Can you work these out from the model? Positions are in its coordinate system, mm. A direction names the side the tool comes from. Round coordinates to 2 decimals unless told otherwise and drop trailing zeros. Order: outer loops, then holes, each group sorted by start corner. A loop starts at its lowest first (then second) coordinate and runs counter-clockwise, first axis right, second up. Notation, with made-up numbers: (57.25, 64.25) -> (109.25, 64.25) arc R27 cw to (109.25, 89.25) -> close; hole circle Ø11 at (21, -15). An arc over 180 degrees is marked (long way). Use a Markdown table: item, result. Add a question column.
Q1. I need wall thicknesses on line 1 along X through (y, z) = (-31, 0.5); line 2 along X through (y, z) = (-40, 1.3); line 3 along Y through (x, z) = (12, 4.1). Which ranges of each line are inside material? Lowest first, please. Write a range as [from, to].
Q2. If we section it at C-C on z = 4.1: Give the number of separate pieces and of enclosed holes in the cut face, plus the area to 3 significant figures.
Q3. I'm going to push flat-ended pins straight in: pin 1 Ø2 at (x, y) = (13, -31.5) entering from -Z; pin 2 Ø1 at (x, y) = (45.5, -13.5) entering from +Z; pin 3 Ø5.5 at (x, y) = (-23, 43) entering from -Z. Where does each tip first touch, or does it pass through?
Q4. We'd pull the mould along Y, two halves only. Please class faces 5 (the face through (-22, 41, 2)), 6 (the face through (-39, -2, 5)), 7 (the face through (13, -4, 3)), 8 (the face through (80.2, 20.06, 2.46)): +Y half, -Y half, draft (parallel to the pull), parting line (faces both ways), or undercut.
Q5. If we section it at D-D on y = -50: List the corners of the cut face in (x, z) for me, plus the area to 3 significant figures.
Q6. If we section it at A-A on y = -26: List the corners of the cut face in (x, z) for me.
Q7. If we section it at B-B on x = 5.5: List the corners of the cut face in (y, z) for me.
Q8. For faces 1 (the face through (24.22, -78.78, 2.46)), 2 (the face through (-68, 18, 3)), 3 (the face through (-34, 71, 3)), 4 (the face through (0, -58, 1.5)), which set-ups out of +Z, -Z, +X, -X, +Y, -Y let a thin tool reach every point of the face, with its end or its side?
```python
from build123d import *

# Parameters (mm, degrees)
EXTRUDE_2156_DEPTH      = 5
FILLET_3_R              = 1.5
FILLET_4_R              = 1.5
FILLET_5_R              = 1.5
FILLET_6_R              = 1.5
FILLET_8_R              = 1.5
FILLET_9_R              = 1.5
FILLET_10_R             = 1
SKETCH_5_R              = 1.5
CUT_EXTRUDE_4477_DEPTH  = 2
SKETCH_12_R             = 3.5
CUT_EXTRUDE_5428_DEPTH  = 3
CUT_EXTRUDE_START       = -3.5
CUT_EXTRUDE_6211_DEPTH  = 3.5
SKETCH_8_W              = 26
SKETCH_8_H              = 49
CUT_EXTRUDE_6713_DEPTH  = 5
SKETCH_9_R              = 1.5
CUT_EXTRUDE_7322_DEPTH  = 2
SKETCH_10_R             = 3.5
CUT_EXTRUDE_8110_DEPTH  = 3
SKETCH_11_R             = 1.5
CUT_EXTRUDE_8691_DEPTH  = 5
SKETCH_14_W             = 68
SKETCH_14_H             = 4
CUT_EXTRUDE_8943_DEPTH  = 10
SKETCH_15_R             = 1
CUT_EXTRUDE_9740_DEPTH  = 4
SKETCH_16_R             = 1
CUT_EXTRUDE_10725_DEPTH = 4
SKETCH_17_R             = 1
CUT_EXTRUDE_11590_DEPTH = 4
SKETCH_18_R             = 3.5
CUT_EXTRUDE_12205_DEPTH = 2
SKETCH_19_W             = 68
SKETCH_19_H             = 11
CUT_EXTRUDE_3_DEPTH     = 5


with BuildPart() as part:
    # 草图1 → Extrude 2156 (new body)
    with BuildSketch(Plane.XY):
        with BuildLine():
            Line((40.572949017, 63.247239682), (56.631189606, 41.14496766))
            Line((56.631189606, 41.14496766), (72.029031786, 19.951656069))
            ThreePointArc((72.029031786, 19.951656069), (73.431066875, 18.895554003), (75.184005217, 18.804663237))
            Line((75.184005217, 18.804663237), (86.825399574, 21.716353029))
            ThreePointArc((86.825399574, 21.716353029), (88.776371499, -11.358074817), (78.561436026, -42.875992928))
            Line((78.561436026, -42.875992928), (68.669508852, -37.477336526))
            ThreePointArc((68.669508852, -37.477336526), (66.987138464, -37.120716922), (65.385340306, -37.74664849))
            Line((65.385340306, -37.74664849), (43.096303273, -55.160752752))
            Line((43.096303273, -55.160752752), (23.649832714, -70.354000687))
            ThreePointArc((23.649832714, -70.354000687), (22.63495231, -71.818183128), (22.6292966, -73.599693854))
            Line((22.6292966, -73.599693854), (26.30288371, -85.547696103))
            ThreePointArc((26.30288371, -85.547696103), (0, -89.5), (-26.30288371, -85.547696103))
            Line((-26.30288371, -85.547696103), (-22.6292966, -73.599693854))
            ThreePointArc((-22.6292966, -73.599693854), (-22.63495231, -71.818183128), (-23.649832714, -70.354000687))
            Line((-23.649832714, -70.354000687), (-43.096303273, -55.160752752))
            Line((-43.096303273, -55.160752752), (-65.385340306, -37.74664849))
            ThreePointArc((-65.385340306, -37.74664849), (-66.987138464, -37.120716922), (-68.669508852, -37.477336526))
            Line((-68.669508852, -37.477336526), (-78.561436026, -42.875992928))
            ThreePointArc((-78.561436026, -42.875992928), (-88.776371499, -11.358074817), (-86.825399574, 21.716353029))
            Line((-86.825399574, 21.716353029), (-75.184005217, 18.804663237))
            ThreePointArc((-75.184005217, 18.804663237), (-73.431066875, 18.895554003), (-72.029031786, 19.951656069))
            Line((-72.029031786, 19.951656069), (-56.631189606, 41.14496766))
            Line((-56.631189606, 41.14496766), (-40.572949017, 63.247239682))
            ThreePointArc((-40.572949017, 63.247239682), (-40.146830451, 64.083544456), (-40, 65.010595439))
            Line((-40, 65.010595439), (-40, 74))
            Line((-40, 74), (-40, 80.06403687))
            Line((-40, 80.06403687), (-34, 82.790397994))
            Line((-34, 82.790397994), (-34, 77))
            Line((-34, 77), (34, 77))
            Line((34, 77), (34, 82.790397994))
            Line((34, 82.790397994), (40, 80.06403687))
            Line((40, 80.06403687), (40, 74))
            Line((40, 74), (40, 65.010595439))
            ThreePointArc((40, 65.010595439), (40.146830451, 64.083544456), (40.572949017, 63.247239682))
        make_face()
    extrude(amount=EXTRUDE_2156_DEPTH)

    # 圆角3
    fillet_3_edges = [part.edges().sort_by_distance(p)[0] for p in [
        (78.561436026, -42.875992928, 2.5),
    ]]
    fillet(fillet_3_edges, radius=FILLET_3_R)

    # 圆角4
    fillet_4_edges = [part.edges().sort_by_distance(p)[0] for p in [
        (26.30288371, -85.547696103, 2.5),
    ]]
    fillet(fillet_4_edges, radius=FILLET_4_R)

    # 圆角5
    fillet_5_edges = [part.edges().sort_by_distance(p)[0] for p in [
        (-26.30288371, -85.547696103, 2.5),
    ]]
    fillet(fillet_5_edges, radius=FILLET_5_R)

    # 圆角6
    fillet_6_edges = [part.edges().sort_by_distance(p)[0] for p in [
        (-78.561436026, -42.875992928, 2.5),
    ]]
    fillet(fillet_6_edges, radius=FILLET_6_R)

    # 圆角8
    fillet_8_edges = [part.edges().sort_by_distance(p)[0] for p in [
        (86.825399574, 21.716353029, 2.5),
    ]]
    fillet(fillet_8_edges, radius=FILLET_8_R)

    # 圆角9
    fillet_9_edges = [part.edges().sort_by_distance(p)[0] for p in [
        (-86.825399574, 21.716353029, 2.5),
    ]]
    fillet(fillet_9_edges, radius=FILLET_9_R)

    # 圆角10
    fillet_10_edges = [part.edges().sort_by_distance(p)[0] for p in [
        (-40, 80.06403687, 2.5),
        (-34, 82.790397994, 2.5),
        (34, 82.790397994, 2.5),
        (40, 80.06403687, 2.5),
    ]]
    fillet(fillet_10_edges, radius=FILLET_10_R)

    # 草图5 → Cut-Extrude 4477 (cut)
    with BuildSketch(Plane.XY.offset(5)):
        with Locations((47.738500848, 48.280798842)):
            Circle(SKETCH_5_R)
        with Locations((68.310984678, 19.965204039)):
            Circle(SKETCH_5_R)
        with Locations(Location((-68.310984678, 19.965204039, 0), (0, 0, 180))):
            Circle(SKETCH_5_R)
        with Locations(Location((-47.738500848, 48.280798842, 0), (0, 0, 180))):
            Circle(SKETCH_5_R)
        with Locations((60.161576933, -38.020845084)):
            Circle(SKETCH_5_R)
        with Locations((32.581200557, -59.56899672)):
            Circle(SKETCH_5_R)
        with Locations(Location((-60.161576933, -38.020845084, 0), (0, 0, 180))):
            Circle(SKETCH_5_R)
        with Locations(Location((-32.581200557, -59.56899672, 0), (0, 0, 180))):
            Circle(SKETCH_5_R)
    extrude(amount=-CUT_EXTRUDE_4477_DEPTH, mode=Mode.SUBTRACT)

    # 草图12 → Cut-Extrude 5428 (cut)
    with BuildSketch(Plane(origin=(0, 0, 0), x_dir=(-1, 0, 0), z_dir=(0, 0, -1))):
        with Locations((47.738500848, 48.280798842)):
            Circle(SKETCH_12_R)
        with Locations((68.310984678, 19.965204039)):
            Circle(SKETCH_12_R)
        with Locations((-68.310984678, 19.965204039)):
            Circle(SKETCH_12_R)
        with Locations((-47.738500848, 48.280798842)):
            Circle(SKETCH_12_R)
        with Locations((32.581200557, -59.56899672)):
            Circle(SKETCH_12_R)
        with Locations((60.161576933, -38.020845084)):
            Circle(SKETCH_12_R)
        with Locations((13.527038551, -115.928745256)):
            Circle(SKETCH_12_R)
        with Locations((-60.161576933, -38.020845084)):
            Circle(SKETCH_12_R)
        with Locations((-32.581200557, -59.56899672)):
            Circle(SKETCH_12_R)
    extrude(amount=-CUT_EXTRUDE_5428_DEPTH, mode=Mode.SUBTRACT)

    # 草图7 → Cut-Extrude 6211 (cut)
    with BuildSketch(Plane.XY.offset(5).offset(CUT_EXTRUDE_START)):
        with BuildLine():
            Line((-8, 77), (-8, -89.141741064))
            ThreePointArc((-8, -89.141741064), (0, -89.5), (8, -89.141741064))
            Line((8, -89.141741064), (8, 77))
            Line((8, 77), (-8, 77))
        make_face()
    extrude(amount=CUT_EXTRUDE_6211_DEPTH, mode=Mode.SUBTRACT)

    # 草图8 → Cut-Extrude 6713 (cut)
    with BuildSketch(Plane.XY.offset(5)):
        with Locations((0, -3.5)):
            Rectangle(SKETCH_8_W, SKETCH_8_H)
    extrude(amount=-CUT_EXTRUDE_6713_DEPTH, mode=Mode.SUBTRACT)

    # 草图9 → Cut-Extrude 7322 (cut)
    with BuildSketch(Plane.XY.offset(5)):
        with Locations((12, 25)):
            Circle(SKETCH_9_R)
        with Locations(Location((-12, 25, 0), (0, 0, 180))):
            Circle(SKETCH_9_R)
        with Locations((-12, -32)):
            Circle(SKETCH_9_R)
        with Locations(Location((12, -32, 0), (0, 0, 180))):
            Circle(SKETCH_9_R)
    extrude(amount=-CUT_EXTRUDE_7322_DEPTH, mode=Mode.SUBTRACT)

    # 草图10 → Cut-Extrude 8110 (cut)
    with BuildSketch(Plane(origin=(0, 0, 0), x_dir=(-1, 0, 0), z_dir=(0, 0, -1))):
        with Locations((12, 25)):
            Circle(SKETCH_10_R)
        with Locations(Location((-12, 25, 0), (0, 0, 180))):
            Circle(SKETCH_10_R)
        with Locations(Location((12, -32, 0), (0, 0, 180))):
            Circle(SKETCH_10_R)
        with Locations((-12, -32)):
            Circle(SKETCH_10_R)
    extrude(amount=-CUT_EXTRUDE_8110_DEPTH, mode=Mode.SUBTRACT)

    # 草图11 → Cut-Extrude 8691 (cut)
    with BuildSketch(Plane.XY.offset(5)):
        with Locations((22.5, 57.8)):
            Circle(SKETCH_11_R)
        with Locations((22.5, 42.8)):
            Circle(SKETCH_11_R)
        with Locations(Location((-22.5, 42.8, 0), (0, 0, 180))):
            Circle(SKETCH_11_R)
        with Locations(Location((-22.5, 57.8, 0), (0, 0, 180))):
            Circle(SKETCH_11_R)
    extrude(amount=-CUT_EXTRUDE_8691_DEPTH, mode=Mode.SUBTRACT)

    # 草图14 → Cut-Extrude 8943 (cut)
    with BuildSketch(Plane(origin=(0, 0, 0), x_dir=(-1, 0, 0), z_dir=(0, 0, -1))):
        with Locations((0, 75)):
            Rectangle(SKETCH_14_W, SKETCH_14_H)
    extrude(amount=-CUT_EXTRUDE_8943_DEPTH, mode=Mode.SUBTRACT)

    # 草图15 → Cut-Extrude 9740 (cut)
    with BuildSketch(Plane.XY.offset(5)):
        with Locations(Location((-45.5, -13.5, 0), (0, 0, 180))):
            Circle(SKETCH_15_R)
        with Locations(Location((-34, 43, 0), (0, 0, 180))):
            Circle(SKETCH_15_R)
        with Locations((34, 43)):
            Circle(SKETCH_15_R)
        with Locations((45.5, -13.5)):
            Circle(SKETCH_15_R)
    extrude(amount=-CUT_EXTRUDE_9740_DEPTH, mode=Mode.SUBTRACT)

    # 草图16 → Cut-Extrude 10725 (cut)
    with BuildSketch(Plane.XY.offset(5)):
        with Locations((-70.6, -32.7)):
            Circle(SKETCH_16_R)
        with Locations((-70.6, 9.5)):
            Circle(SKETCH_16_R)
        with Locations((70.6, 9.5)):
            Circle(SKETCH_16_R)
        with Locations((70.6, -32.7)):
            Circle(SKETCH_16_R)
    extrude(amount=-CUT_EXTRUDE_10725_DEPTH, mode=Mode.SUBTRACT)

    # 草图17 → Cut-Extrude 11590 (cut)
    with BuildSketch(Plane.XY.offset(5)):
        with Locations((85.690046638, -3.237648509)):
            Circle(SKETCH_17_R)
        with Locations((85.690046638, -13.762351491)):
            Circle(SKETCH_17_R)
        with Locations((52.309953362, -13.762351491)):
            Circle(SKETCH_17_R)
        with Locations((52.309953362, -3.237648509)):
            Circle(SKETCH_17_R)
        with Locations(Location((-52.309953362, -13.762351491, 0), (0, 0, 180))):
            Circle(SKETCH_17_R)
        with Locations(Location((-85.690046638, -3.237648509, 0), (0, 0, 180))):
            Circle(SKETCH_17_R)
        with Locations(Location((-52.309953362, -3.237648509, 0), (0, 0, 180))):
            Circle(SKETCH_17_R)
        with Locations(Location((-85.690046638, -13.762351491, 0), (0, 0, 180))):
            Circle(SKETCH_17_R)
    extrude(amount=-CUT_EXTRUDE_11590_DEPTH, mode=Mode.SUBTRACT)

    # 草图18 → Cut-Extrude 12205 (cut)
    with BuildSketch(Plane(origin=(0, 0, 0), x_dir=(-1, 0, 0), z_dir=(0, 0, -1))):
        with Locations((-22.5, 57.8)):
            Circle(SKETCH_18_R)
        with Locations((-22.5, 42.8)):
            Circle(SKETCH_18_R)
        with Locations((22.5, 42.8)):
            Circle(SKETCH_18_R)
        with Locations((22.5, 57.8)):
            Circle(SKETCH_18_R)
    extrude(amount=-CUT_EXTRUDE_12205_DEPTH, mode=Mode.SUBTRACT)

    # 草图19 → 切除-拉伸3 (cut, symmetric)
    with BuildSketch(Plane.XY.offset(5)):
        with Locations((0, 67.5)):
            Rectangle(SKETCH_19_W, SKETCH_19_H)
    extrude(amount=CUT_EXTRUDE_3_DEPTH, both=True, mode=Mode.SUBTRACT)


solid = part.part
```
Answer below:
| question | item | result |
|---|---|---|
| 1 | line 1 | [-83.96, -15.35], [-8.65, 8.65], [15.35, 83.96] |
| 1 | line 2 | [-80.06, -73.29], [-57.27, 57.27], [73.29, 80.06] |
| 1 | line 3 | [-88.69, -33.5], [-30.5, -28], [21, 23.5], [26.5, 62] |
| 2 | separate pieces | 2 |
| 2 | enclosed holes | 32 |
| 2 | area | 15,900 mm² |
| 3 | pin 1 | z = 3 |
| 3 | pin 2 | z = 1 |
| 3 | pin 3 | z = 2 |
| 4 | face 5 | undercut |
| 4 | face 6 | draft |
| 4 | face 7 | undercut |
| 4 | face 8 | +Y half |
| 5 | outline | (-49.7, 0) -> (49.7, 0) -> (49.7, 5) -> (8, 5) -> (8, 1.5) -> (-8, 1.5) -> (-8, 5) -> (-49.7, 5) -> close |
| 5 | area | 441 mm² |
| 6 | outline | (-85.64, 0) -> (-13, 0) -> (-13, 5) -> (-85.64, 5) -> close; (13, 0) -> (85.64, 0) -> (85.64, 5) -> (13, 5) -> close |
| 7 | outline | (-89.33, 0) -> (-28, 0) -> (-28, 1.5) -> (-89.33, 1.5) -> close; (21, 0) -> (62, 0) -> (62, 1.5) -> (21, 1.5) -> close |
| 8 | face 1 | +Z, -Z, +X |
| 8 | face 2 | -Z |
| 8 | face 3 | +Z, -Z, +Y |
| 8 | face 4 | +Z, +Y, -Y |
